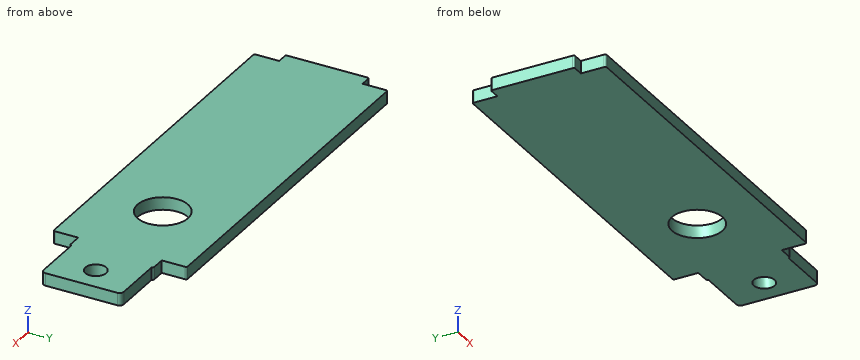
from build123d import *

# Parameters (mm, degrees)
SKETCH1_R          = 3.025
BASE_FLANGE1_DEPTH = 1.5
SKETCH6_R          = 1.25
TAB1_DEPTH         = 1.5


# Sheet-metal steps are written as plain solids
with BuildPart() as part:
    # Sketch1 → Base-Flange1 (new body)
    with BuildSketch(Plane.XY):
        with BuildLine():
            Line((1.4, 17.8), (1.4, 15))
            Line((1.4, 15), (0.2, 15))
            ThreePointArc((0.2, 15), (0.058578644, 14.941421356), (0, 14.8))
            Line((0, 14.8), (0, 5.2))
            ThreePointArc((0, 5.2), (0.058578644, 5.058578644), (0.2, 5))
            Line((0.2, 5), (1.4, 5))
            Line((1.4, 5), (1.4, 2.2))
            ThreePointArc((1.4, 2.2), (1.458578644, 2.058578644), (1.6, 2))
            Line((1.6, 2), (44.4, 2))
            ThreePointArc((44.4, 2), (44.541421356, 2.058578644), (44.6, 2.2))
            Line((44.6, 2.2), (44.6, 5))
            Line((44.6, 5), (46.2, 5))
            ThreePointArc((46.2, 5), (46.341421356, 5.058578644), (46.4, 5.2))
            Line((46.4, 5.2), (46.4, 14.8))
            ThreePointArc((46.4, 14.8), (46.341421356, 14.941421356), (46.2, 15))
            Line((46.2, 15), (44.6, 15))
            Line((44.6, 15), (44.6, 17.8))
            ThreePointArc((44.6, 17.8), (44.541421356, 17.941421356), (44.4, 18))
            Line((44.4, 18), (1.6, 18))
            ThreePointArc((1.6, 18), (1.458578644, 17.941421356), (1.4, 17.8))
        make_face()
        with Locations((35.4, 10)):
            Circle(SKETCH1_R, mode=Mode.SUBTRACT)
    extrude(amount=-BASE_FLANGE1_DEPTH)

    # Sketch6 → Tab1 (add)
    with BuildSketch(Plane.XY):
        with BuildLine():
            Line((46.4, 14.8), (52.4, 14.8))
            ThreePointArc((52.4, 14.8), (52.753553391, 14.653553391), (52.9, 14.3))
            Line((52.9, 14.3), (52.9, 5.7))
            ThreePointArc((52.9, 5.7), (52.753553391, 5.346446609), (52.4, 5.2))
            Line((52.4, 5.2), (46.4, 5.2))
            Line((46.4, 5.2), (46.4, 14.8))
        make_face()
        with Locations((49.8, 10)):
            Circle(SKETCH6_R, mode=Mode.SUBTRACT)
    extrude(amount=-TAB1_DEPTH)


solid = part.part
Could you check a few things on this model? Use its own coordinates, in mm. Give positions to 0.01 mm unless a question says otherwise; leave off trailing zeros. Order: outer loops, then holes, each group sorted by start corner. A loop starts at its lowest first (then second) coordinate and runs counter-clockwise, first axis right, second up. Notation, with made-up numbers: (12.5, 0.5) - (16.5, 0.5) arc R23 cw to (16.5, 27.5) - close; hole circle Ø10 at (-36, 62.25). An arc over 180 degrees is marked (long way). One line per question, with ' | ' between items. Start each with the question number.
Item 1: I want a section at A-A on x = 35.4. Write out the boundary of the cut face in (y, z) (3 decimals).
Item 2: I want a section at D-D on y = 16.75. Write out the boundary of the cut face in (x, z).
Item 3: I'm going to push flat-ended pins straight in: pin 1 Ø8 at (x, y) = (30, 13) entering from +Z; pin 2 Ø5 at (x, y) = (35.4, 10) entering from +Z. Where does each tip first touch, or does it pass through?
Item 4: I want a section at C-C on y = 10. Write out the boundary of the cut face in (x, z) (3 decimals), then the cut area to 3 significant figures.
Item 5: I need wall thicknesses on probe 1 along Y at (x, z) = (49.8, -1.2); probe 2 along X at (y, z) = (9, -0.9); probe 3 along X at (y, z) = (9.25, -1.05). Which ranges of each line are inside material? Lowest first, please. Write a range as [from, to].
Item 6: I want a section at B-B on z = -0.65. Write out the boundary of the cut face in (x, y) (3 decimals).
Verdict:
1) outline: (2, -1.5) - (6.975, -1.5) - (6.975, 0) - (2, 0) - close; (13.025, -1.5) - (18, -1.5) - (18, 0) - (13.025, 0) - close
2) outline: (1.4, -1.5) - (44.6, -1.5) - (44.6, 0) - (1.4, 0) - close
3) pin 1: z = 0 | pin 2: through
4) outline: (0, -1.5) - (32.375, -1.5) - (32.375, 0) - (0, 0) - close; (38.425, -1.5) - (48.55, -1.5) - (48.55, 0) - (38.425, 0) - close; (51.05, -1.5) - (52.9, -1.5) - (52.9, 0) - (51.05, 0) - close | area: 66.5 mm^2
5) probe 1: [5.2, 8.75], [11.25, 14.8] | probe 2: [0, 32.55], [38.25, 49.05], [50.55, 52.9] | probe 3: [0, 32.47], [38.33, 48.8], [50.8, 52.9]
6) outline: (0, 5.2) arc R0.2 ccw to (0.2, 5) - (1.4, 5) - (1.4, 2.2) arc R0.2 ccw to (1.6, 2) - (44.4, 2) arc R0.2 ccw to (44.6, 2.2) - (44.6, 5) - (46.2, 5) arc R0.2 ccw to (46.4, 5.2) - (52.4, 5.2) arc R0.5 ccw to (52.9, 5.7) - (52.9, 14.3) arc R0.5 ccw to (52.4, 14.8) - (46.4, 14.8) arc R0.2 ccw to (46.2, 15) - (44.6, 15) - (44.6, 17.8) arc R0.2 ccw to (44.4, 18) - (1.6, 18) arc R0.2 ccw to (1.4, 17.8) - (1.4, 15) - (0.2, 15) arc R0.2 ccw to (0, 14.8) - close; hole circle Ø6.05 at (35.4, 10); hole circle Ø2.5 at (49.8, 10)
